Verification items for the finished model (mm, model axes). A direction names the side the tool comes from. Round coordinates to 2 decimals unless told otherwise and drop trailing zeros. Write each loop counter-clockwise with the first axis right and the second up, starting at its lowest first coordinate (ties: lowest second). Pieces come first, ordered by that corner, then holes.
from build123d import *

# Parameters (mm, degrees)
F1_DEPTH = 32


with BuildPart() as f1:
    # F0 (on Top) → F1 (new body)
    with BuildSketch(Plane.XY):
        with BuildLine():
            Line((0, 30.1567251716), (0, 0))
            Line((0, 0), (35.1581014693, 0))
            Line((35.1581014693, 0), (35.1581014693, 34.1453179717))
            Line((35.1581014693, 34.1453179717), (5.5145962808, 34.1453179717))
            ThreePointArc((5.5145962808, 34.1453179717), (6.8391912962, 32.7926703645), (7.3227977475, 30.9622790664))
            ThreePointArc((7.3227977475, 30.9622790664), (4.0222975699, 27.2787928126), (0, 30.1567251716))
        make_face()
        with BuildLine():
            ThreePointArc((0, 31.7678329612), (-0.0886160044, 30.9622790664), (0, 30.1567251716))
            Line((0, 30.1567251716), (0, 31.7678329612))
        make_face()
        with BuildLine():
            Line((0, 31.7678329612), (0, 30.1567251716))
            ThreePointArc((0, 30.1567251716), (4.0222975699, 27.2787928126), (7.3227977475, 30.9622790664))
            ThreePointArc((7.3227977475, 30.9622790664), (6.8391912962, 32.7926703645), (5.5145962808, 34.1453179717))
            Line((5.5145962808, 34.1453179717), (1.7195854623, 34.1453179717))
            ThreePointArc((1.7195854623, 34.1453179717), (0.6144583967, 33.1340206882), (0, 31.7678329612))
        make_face()
        with BuildLine():
            Line((0, 34.1453179717), (0, 31.7678329612))
            ThreePointArc((0, 31.7678329612), (0.6144583967, 33.1340206882), (1.7195854623, 34.1453179717))
            Line((1.7195854623, 34.1453179717), (0, 34.1453179717))
        make_face()
        with BuildLine():
            Line((1.7195854623, 34.1453179717), (5.5145962808, 34.1453179717))
            ThreePointArc((5.5145962808, 34.1453179717), (3.6170908716, 34.6679859424), (1.7195854623, 34.1453179717))
        make_face()
    extrude(amount=F1_DEPTH)


solid = f1.part
Q1. Material ranges on line 1 along Y through (x, z) = (20, 15); line 2 along X through (y, z) = (30, 17); line 3 along Y through (x, z) = (2, 14), recorded low to high.
Recorded:
line 1: y = 0 to 34.15
line 2: x = 0 to 35.16
line 3: y = 0 to 34.3
Q2. Sectioned sample at A-A (z = 18.5). Enter the section's corners in (x, y), plus the area to 3 significant figures.
Recorded:
outline: (0, 0) - (35.16, 0) - (35.16, 34.15) - (5.51, 34.15) arc R3.71 ccw to (1.72, 34.15) - (0, 34.15) - (0, 31.77) arc R3.71 ccw to (0, 30.16) - close
area: 1,200 mm2
Q3. Sectioned sample at B-B (x = 16.5). Enter the section's corners in (y, z).
Recorded:
outline: (0, 0) - (34.15, 0) - (34.15, 32) - (0, 32) - close
Q4. Depth check by flat-ended pin: P1, Ø1.2, axis at y = 33.5, z = 15, coming from the -X side; P2, Ø12, axis at x = 10, z = 5.5, coming from the +Y side; P3, Ø6, axis at x = 10, z = 14, coming from the +Y side. Enter the tip coordinate at first touch or a pass-through.
Recorded:
P1: stops at x = 0
P2: stops at y = 34.65
P3: stops at y = 34.15
Q5. Tool access check on faces 1 (the flat face through (0, 15, 16)), 2 (the flat face through (21, 34.145, 16)), 3 (the flat face through (0, 33, 16)), 4 (the cylindrical face through (-0.09, 30.97, 15.78)), 5 (the cylindrical face through (3.645, 34.668, 15.776)). Record the directions out of +Z, -Z, +X, -X, +Y, -Y that give a thin tool (end or side, any length) a straight path to the whole face; none if there is none.
Recorded:
face 1: +Z, -Z, -X, -Y
face 2: +Z, -Z, +X, +Y
face 3: +Z, -Z, -X, +Y
face 4: +Z, -Z, -X
face 5: +Z, -Z, +Y
